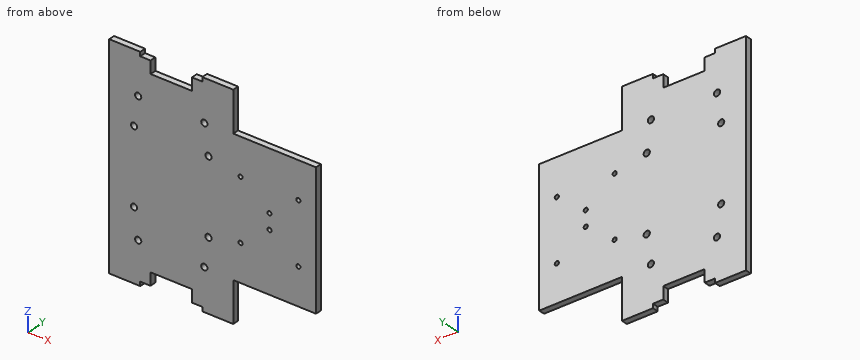
from build123d import *

# Parameters (mm, degrees)
SKETCH_1_R      = 1
SKETCH_1_R_2    = 1.5
EXTRUDE_1_DEPTH = 2.95


with BuildPart() as part:
    # 草图1 → 凸台-拉伸1 (new body)
    with BuildSketch(Plane(origin=(0, 0, 0), x_dir=(1, 0, 0), z_dir=(0, 1, 0))):
        Polygon((25, 50), (20, 50), (20, 44), (0, 44), (0, 50), (-5, 50), (-5, 52), (-20, 52), (-20, 50), (-20, -50), (-20, -52), (-5, -52), (-5, -50), (0, -50), (0, -44), (20, -44), (20, -50), (25, -50), (25, -52), (40, -52), (40, -50), (40, -32.5), (70, -32.5), (80, -32.5), (80, -30), (80, 30), (80, 32.5), (70, 32.5), (40, 32.5), (40, 50), (40, 52), (25, 52), align=None)
        with Locations(Location((71.5, 14.7, 0), (0, 0, 90))):
            Circle(SKETCH_1_R, mode=Mode.SUBTRACT)
        with Locations(Location((43.5, 14.7, 0), (0, 0, 90))):
            Circle(SKETCH_1_R, mode=Mode.SUBTRACT)
        with Locations(Location((57.5, 3.7, 0), (0, 0, 90))):
            Circle(SKETCH_1_R, mode=Mode.SUBTRACT)
        with Locations(Location((26, 32, 0), (0, 0, 270))):
            Circle(SKETCH_1_R_2, mode=Mode.SUBTRACT)
        with Locations(Location((-6, 32, 0), (0, 0, 270))):
            Circle(SKETCH_1_R_2, mode=Mode.SUBTRACT)
        with Locations(Location((28, 18, 0), (0, 0, 270))):
            Circle(SKETCH_1_R_2, mode=Mode.SUBTRACT)
        with Locations(Location((-8, 18, 0), (0, 0, 270))):
            Circle(SKETCH_1_R_2, mode=Mode.SUBTRACT)
        with Locations(Location((-8, -18, 0), (0, 0, 90))):
            Circle(SKETCH_1_R_2, mode=Mode.SUBTRACT)
        with Locations(Location((28, -18, 0), (0, 0, 90))):
            Circle(SKETCH_1_R_2, mode=Mode.SUBTRACT)
        with Locations(Location((-6, -32, 0), (0, 0, 90))):
            Circle(SKETCH_1_R_2, mode=Mode.SUBTRACT)
        with Locations(Location((26, -32, 0), (0, 0, 90))):
            Circle(SKETCH_1_R_2, mode=Mode.SUBTRACT)
        with Locations(Location((57.5, -3.7, 0), (0, 0, 270))):
            Circle(SKETCH_1_R, mode=Mode.SUBTRACT)
        with Locations(Location((43.5, -14.7, 0), (0, 0, 270))):
            Circle(SKETCH_1_R, mode=Mode.SUBTRACT)
        with Locations(Location((71.5, -14.7, 0), (0, 0, 270))):
            Circle(SKETCH_1_R, mode=Mode.SUBTRACT)
    extrude(amount=EXTRUDE_1_DEPTH)


solid = part.part
Verification items for the finished model (mm, model axes). Give positions to 0.01 mm unless a question says otherwise; leave off trailing zeros. Loops run counter-clockwise (first coordinate to the right, second up) from the corner with the lowest first, then second, coordinate; pieces in that order, holes last.
1) Depth check by flat-ended pin: pin 1 Ø0.9 at (x, y) = (8, 1.5) entering from -Z; pin 2 Ø0.9 at (x, y) = (60.5, 1) entering from -Z; pin 3 Ø2.5 at (x, z) = (-6, 32) entering from -Y; pin 4 Ø0.9 at (x, y) = (23, 1) entering from -Z. Enter the tip coordinate at first touch or a pass-through.
2) Thickness scan on line 1 along Z through (x, y) = (71.5, 1.55); line 2 along X through (y, z) = (1.45, 32); line 3 along X through (y, z) = (2.2, -18). Record the ranges inside material, lowest first.
3) Sectioned sample at A-A, the plane z = -18. Enter the section's corners in (x, y), then the cut area to 3 significant figures.
4) Sectioned sample at B-B, the plane z = 46. Enter the section's corners in (x, y).
5) Sectioned sample at C-C, the plane y = 0.6. Count the separate pieces of the cut face and the enclosed holes in it, then the cut area to 3 significant figures.
6) Sectioned sample at D-D, the plane x = 16.5. Enter the section's corners in (y, z).
Answers:
1. pin 1: stops at z = -44
1. pin 2: stops at z = -32.5
1. pin 3: passes through
1. pin 4: stops at z = -50
2. line 1: z = -32.5 to -15.7, -13.7 to 13.7, 15.7 to 32.5
2. line 2: x = -20 to -7.5, -4.5 to 24.5, 27.5 to 80
2. line 3: x = -20 to -9.5, -6.5 to 26.5, 29.5 to 80
3. outline: (-20, 0) - (-9.5, 0) - (-9.5, 2.95) - (-20, 2.95) - close; (-6.5, 0) - (26.5, 0) - (26.5, 2.95) - (-6.5, 2.95) - close; (29.5, 0) - (80, 0) - (80, 2.95) - (29.5, 2.95) - close
3. area: 277 mm2
4. outline: (-20, 0) - (0, 0) - (0, 2.95) - (-20, 2.95) - close; (20, 0) - (40, 0) - (40, 2.95) - (20, 2.95) - close
5. separate pieces: 1
5. enclosed holes: 14
5. area: 8,400 mm2
6. outline: (0, -44) - (2.95, -44) - (2.95, 44) - (0, 44) - close
